Geometry: final body of the model. Coordinates: model frame, mm. Face numbers are marked on the shaded views. A direction names the side the tool comes from. Give positions to 0.01 mm unless a question says otherwise; leave off trailing zeros. Loops run counter-clockwise (first coordinate to the right, second up) from the corner with the lowest first, then second, coordinate; pieces in that order, holes last. Notation, with made-up numbers: (-7.75, -23) - (41.25, -23) arc R11 ccw to (41.25, -3) - close; hole circle Ø4 at (34.25, 77). An arc over 180 degrees is marked (long way). Answer in a Markdown table with one row per item.
from build123d import *

# Parameters (mm, degrees)
BOSS_EXTRUDE1_DEPTH = 16
SKETCH14_R          = 1.5
CUT_EXTRUDE13_DEPTH = 50
FILLET1_R           = 10


with BuildPart() as part:
    # Sketch7 → Boss-Extrude1 (new body)
    with BuildSketch(Plane.XY):
        Polygon((9.868798372, -27.16601268), (9.868798372, -22.16601268), (-2.131201628, -22.16601268), (-2.131201628, -27.16601268), (-8.131201628, -27.16601268), (-21.131201628, -27.16601268), (-21.131201628, -22.16601268), (-11.131201628, -22.16601268), (-11.131201628, -17.16601268), (18.868798372, -17.16601268), (18.868798372, -22.16601268), (28.868798372, -22.16601268), (28.868798372, -27.16601268), (15.868798372, -27.16601268), align=None)
    extrude(amount=BOSS_EXTRUDE1_DEPTH)

    # Sketch14 → Cut-Extrude13 (cut)
    with BuildSketch(Plane(origin=(0, -27.16601268, 0), x_dir=(1, 0, 0), z_dir=(0, 1, 0))):
        with Locations(Location((-18.631201628, -3, 0), (0, 0, 90))):
            Circle(SKETCH14_R)
        with Locations(Location((-18.631201628, -13, 0), (0, 0, 90))):
            Circle(SKETCH14_R)
        with Locations(Location((26.368798372, -3, 0), (0, 0, 270))):
            Circle(SKETCH14_R)
        with Locations(Location((26.368798372, -13, 0), (0, 0, 270))):
            Circle(SKETCH14_R)
    extrude(amount=CUT_EXTRUDE13_DEPTH, mode=Mode.SUBTRACT)

    # Fillet1
    # the kernel refuses this fillet: 10 mm, written as the material it takes off along each edge
    with BuildSketch(Plane(origin=(-11.131201628, -17.16601268, -21.650635095), x_dir=(0, -1, 0), z_dir=(0, 0, 1))) as fillet1_piece_1:
        with BuildLine():
            CenterArc((10, 8.660254038), FILLET1_R, 180, 60)
            Line((0, 8.660254038), (-0.2, 8.660254038))
            Line((-0.2, 8.660254038), (-0.2, 0))
            Line((-0.2, 0), (0, -0.2))
            ThreePointArc((0, -0.2), (2.5, -0.2), (4.9, -0.173205081))
            Line((4.9, -0.173205081), (5, 0))
        make_face()
    extrude(amount=59.301270189, mode=Mode.SUBTRACT)
    with BuildSketch(Plane(origin=(18.868798372, -17.16601268, -21.650635095), x_dir=(-1, 0, 0), z_dir=(0, 0, 1))) as fillet1_piece_2:
        with BuildLine():
            CenterArc((8.660254038, 10), FILLET1_R, 210, 60)
            Line((0, 5), (-0.173205081, 4.9))
            ThreePointArc((-0.173205081, 4.9), (-0.2, 2.5), (-0.2, 0))
            Line((-0.2, 0), (0, -0.2))
            Line((0, -0.2), (8.660254038, -0.2))
            Line((8.660254038, -0.2), (8.660254038, 0))
        make_face()
    extrude(amount=59.301270189, mode=Mode.SUBTRACT)


solid = part.part
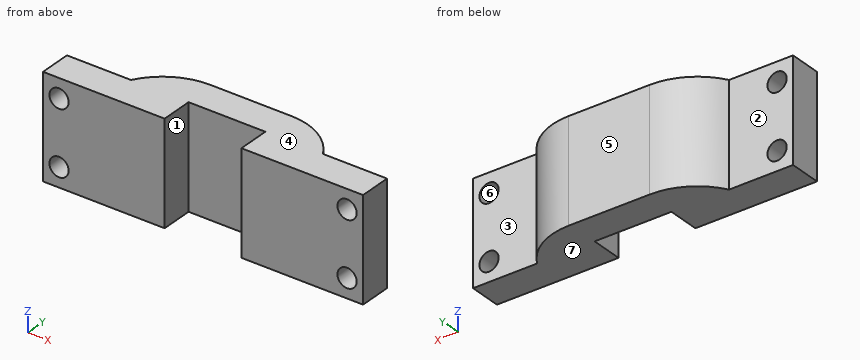
Q1. Reachability of the marked faces 1, 2 and 3 from +Z, -Z, +X, -X, +Y, -Y: full face, straight path, thin tool, end or side. Return the list, or none.
Check values:
| item | result |
|---|---|
| face 1 | +Z, -Z, -Y |
| face 2 | +Z, -Z, -X, +Y |
| face 3 | +Z, -Z, +X, +Y |
Q2. First-contact query: pin 1 (3.5 mm diameter, centred on x = 26.37, z = 3, fed in from +Y); pin 2 (9.5 mm diameter, centred on x = 3.5, z = 7.5, fed in from -Y); pin 3 (2 mm diameter, centred on y = -20.5, z = 13, fed in from -X). Flat tips, straight axial feed; report the tip coordinate or a pass-through.
Check values:
| item | result |
|---|---|
| pin 1 | y = -22.17 |
| pin 2 | y = -22.17 |
| pin 3 | x = -10.71 |
Q3. Material intervals for line 1 along X through (y, z) = (-25, 13); line 2 along X through (y, z) = (-24.5, 8.5); line 3 along X through (y, z) = (-22.25, 13.5), sorted ascending.
Check values:
| item | result |
|---|---|
| line 1 | -21.13 to -20.13, -17.13 to -2.13, 9.87 to 24.87, 27.87 to 28.87 |
| line 2 | -21.13 to -2.13, 9.87 to 28.87 |
| line 3 | -21.13 to -20.05, -17.22 to -2.13, 9.87 to 24.95, 27.78 to 28.87 |
Q4. Cut plane B-B (y = -25.5). Output: boundary loops of the cut face in (x, z).
Check values:
| item | result |
|---|---|
| outline | (-21.13, 0) - (-2.13, 0) - (-2.13, 16) - (-21.13, 16) - close; (9.87, 0) - (28.87, 0) - (28.87, 16) - (9.87, 16) - close; hole circle Ø3 at (-18.63, 3); hole circle Ø3 at (-18.63, 13); hole circle Ø3 at (26.37, 3); hole circle Ø3 at (26.37, 13) |
Q5. Cut plane D-D (x = -14). Output: boundary loops of the cut face in (y, z), and give its area (3 significant figures).
Check values:
| item | result |
|---|---|
| outline | (-27.17, 0) - (-22.17, 0) - (-22.17, 16) - (-27.17, 16) - close |
| area | 80.0 mm² |
Q6. Cut plane A-A (z = 3). Output: boundary loops of the cut face in (x, y).
Check values:
| item | result |
|---|---|
| outline | (-21.13, -27.17) - (-20.13, -27.17) - (-20.13, -22.17) - (-21.13, -22.17) - close; (-17.13, -27.17) - (-2.13, -27.17) - (-2.13, -22.17) - (9.87, -22.17) - (9.87, -27.17) - (24.87, -27.17) - (24.87, -22.17) - (18.87, -22.17) arc R10 ccw to (10.21, -17.17) - (-2.47, -17.17) arc R10 ccw to (-11.13, -22.17) - (-17.13, -22.17) - close; (27.87, -27.17) - (28.87, -27.17) - (28.87, -22.17) - (27.87, -22.17) - close |
Q7. Cut plane C-C (z = 7.25). Output: boundary loops of the cut face in (x, y).
Check values:
| item | result |
|---|---|
| outline | (-21.13, -27.17) - (-2.13, -27.17) - (-2.13, -22.17) - (9.87, -22.17) - (9.87, -27.17) - (28.87, -27.17) - (28.87, -22.17) - (18.87, -22.17) arc R10 ccw to (10.21, -17.17) - (-2.47, -17.17) arc R10 ccw to (-11.13, -22.17) - (-21.13, -22.17) - close |
Q8. Draft query along Z for the marked faces 4, 5, 6 and 7. Return one class per face: pulls with the +Z half, pulls with the -Z half, needs draft (parallel to the pull), parting line crosses it, or undercut.
Check values:
| item | result |
|---|---|
| face 4 | pulls with the +Z half |
| face 5 | needs draft |
| face 6 | undercut |
| face 7 | pulls with the -Z half |
